```python
from build123d import *

# Parameters (mm, degrees)
CROQUIS1_R                                           = 3
CROQUIS1_R_2                                         = 3.25
CROQUIS1_W                                           = 26.6
CROQUIS1_H                                           = 16
CROQUIS1_W_2                                         = 31
CROQUIS1_W_3                                         = 35.15
SALIENTE_EXTRUIR1_DEPTH                              = 8
REDONDEO3_R                                          = 5
AVELLANADO_PARA_TORNILLO_CON_CABEZA_OVAL_D           = 4.4958
AVELLANADO_PARA_TORNILLO_CON_CABEZA_OVAL_CSINK_D     = 8.4328
AVELLANADO_PARA_TORNILLO_CON_CABEZA_OVAL_CSINK_ANGLE = 82


with BuildPart() as part:
    # Croquis1 → Saliente-Extruir1 (new body)
    with BuildSketch(Plane(origin=(0, 0, 0), x_dir=(1, 0, 0), z_dir=(0, 1, 0))):
        with BuildLine():
            Line((0, -50.075), (0, 50.075))
            Line((0, 50.075), (8.85, 50.075))
            ThreePointArc((8.85, 50.075), (16.027133829, 47.102133829), (19, 39.925))
            Line((19, 39.925), (19, 31.15))
            ThreePointArc((19, 31.15), (20.757359313, 26.907359313), (25, 25.15))
            Line((25, 25.15), (136.6, 25.15))
            ThreePointArc((136.6, 25.15), (140.842640687, 26.907359313), (142.6, 31.15))
            Line((142.6, 31.15), (142.6, 69.675))
            ThreePointArc((142.6, 69.675), (152.6, 79.675), (162.6, 69.675))
            Line((162.6, 69.675), (162.6, -69.675))
            ThreePointArc((162.6, -69.675), (152.6, -79.675), (142.6, -69.675))
            Line((142.6, -69.675), (142.6, -31.15))
            ThreePointArc((142.6, -31.15), (140.842640687, -26.907359313), (136.6, -25.15))
            Line((136.6, -25.15), (25, -25.15))
            ThreePointArc((25, -25.15), (20.757359313, -26.907359313), (19, -31.15))
            Line((19, -31.15), (19, -39.925))
            ThreePointArc((19, -39.925), (16.027133829, -47.102133829), (8.85, -50.075))
            Line((8.85, -50.075), (0, -50.075))
        make_face()
        with Locations(Location((152.6, 69.675, 0), (0, 0, 270))):
            Circle(CROQUIS1_R, mode=Mode.SUBTRACT)
        with Locations(Location((152.6, -69.675, 0), (0, 0, 270))):
            Circle(CROQUIS1_R, mode=Mode.SUBTRACT)
        with Locations(Location((8.85, 39.925, 0), (0, 0, 270))):
            Circle(CROQUIS1_R_2, mode=Mode.SUBTRACT)
        with Locations(Location((8.85, -39.925, 0), (0, 0, 90))):
            Circle(CROQUIS1_R_2, mode=Mode.SUBTRACT)
        with Locations((137.3, 0)):
            Rectangle(CROQUIS1_W, CROQUIS1_H, mode=Mode.SUBTRACT)
        with Locations((99, 0)):
            Rectangle(CROQUIS1_W_2, CROQUIS1_H, mode=Mode.SUBTRACT)
        with Locations((43.575, 0)):
            Rectangle(CROQUIS1_W_3, CROQUIS1_H, mode=Mode.SUBTRACT)
    extrude(amount=SALIENTE_EXTRUIR1_DEPTH)

    # Redondeo3
    redondeo3_edges = [part.edges().sort_by_distance(p)[0] for p in [
        (83.5, 4, -8),
        (83.5, 4, 8),
        (114.5, 4, 8),
        (114.5, 4, -8),
        (124, 4, -8),
        (124, 4, 8),
        (150.6, 4, 8),
        (150.6, 4, -8),
        (26, 4, -8),
        (26, 4, 8),
        (61.15, 4, 8),
        (61.15, 4, -8),
    ]]
    fillet(redondeo3_edges, radius=REDONDEO3_R)

    # Avellanado para tornillo con cabeza ovalada de #81 (through all)
    with Locations(Plane(origin=(0, 8, 0), x_dir=(1, 0, 0), z_dir=(0, 1, 0))):
        with Locations((74.55, 20.5), (129.65, 20.5), (74.55, -20.5), (129.65, -20.5)):
            CounterSinkHole(AVELLANADO_PARA_TORNILLO_CON_CABEZA_OVAL_D / 2, AVELLANADO_PARA_TORNILLO_CON_CABEZA_OVAL_CSINK_D / 2, counter_sink_angle=AVELLANADO_PARA_TORNILLO_CON_CABEZA_OVAL_CSINK_ANGLE)


solid = part.part
```
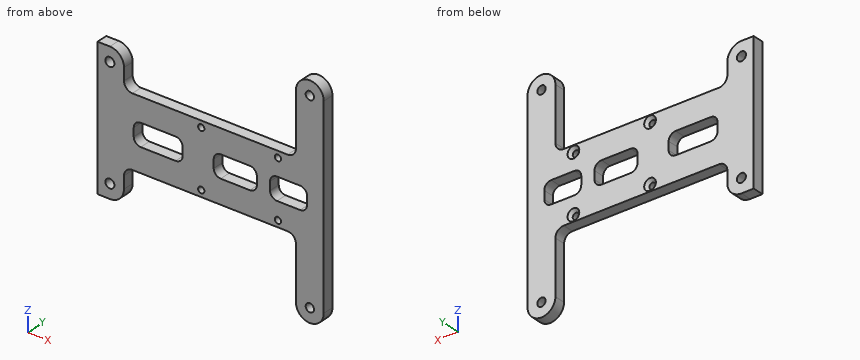
Geometry: final body of the model. Coordinates: model frame, mm. Round coordinates to 2 decimals unless told otherwise and drop trailing zeros. Order: outer loops, then holes, each group sorted by start corner. A loop starts at its lowest first (then second) coordinate and runs counter-clockwise, first axis right, second up. Notation, with made-up numbers: M -34,80.5 L -22,80.5 A19 ccw -22,97.5 Z; hole C 62,-15 d4. An arc over 180 degrees is marked long. One line per item, written item: value.
(1) Cut plane A-A (x = 152.6). Return the cut outline in (y, z) (3 decimals).
Result sheet:
outline: M 0,-79.675 L 8,-79.675 L 8,-72.675 L 0,-72.675 Z; M 0,-66.675 L 8,-66.675 L 8,66.675 L 0,66.675 Z; M 0,72.675 L 8,72.675 L 8,79.675 L 0,79.675 Z
(2) Cut plane B-B (z = 20.5). Return the cut outline in (x, y), and give its area (3 significant figures).
Result sheet:
outline: M 0,0 L 72.3,0 L 72.3,5.74 L 70.33,8 L 0,8 Z; M 76.8,0 L 127.4,0 L 127.4,5.74 L 125.43,8 L 78.77,8 L 76.8,5.74 Z; M 131.9,0 L 162.6,0 L 162.6,8 L 133.87,8 L 131.9,5.74 Z
area: 1,220 mm2
(3) Cut plane D-D (x = 74.55). Return the cut outline in (y, z).
Result sheet:
outline: M 0,-25.15 L 8,-25.15 L 8,-24.72 L 5.74,-22.75 L 0,-22.75 Z; M 0,-18.25 L 5.74,-18.25 L 8,-16.28 L 8,16.28 L 5.74,18.25 L 0,18.25 Z; M 0,22.75 L 5.74,22.75 L 8,24.72 L 8,25.15 L 0,25.15 Z
(4) Line query: probe 1 along X at (y, z) = (1.75, 1.5); probe 2 along X at (y, z) = (3.3, -20.5); probe 3 along Z at (x, y) = (129.65, 1.8). Output: solid intervals per line, ascending. Write a range as [from, to].
Result sheet:
probe 1: [0, 26], [61.15, 83.5], [114.5, 124], [150.6, 162.6]
probe 2: [0, 72.3], [76.8, 127.4], [131.9, 162.6]
probe 3: [-25.15, -22.75], [-18.25, -8], [8, 18.25], [22.75, 25.15]
(5) Pin query (flat end, axial travel): P1, Ø2.5, axis at x = 102.5, y = 3, coming from the +Z side; P2, Ø4, axis at x = 47, y = 5.5, coming from the -Z side. Return the tip coordinate at first contact, or that it passes through.
Result sheet:
P1: z = 25.15
P2: z = -25.15
(6) Cut plane C-C (y = 3.25). Give the number of separate pieces and of enclosed holes in the cut face, and give its area (3 significant figures).
Result sheet:
separate pieces: 1
enclosed holes: 11
area: 9,600 mm2
